Here's how the part is built. I have some questions about the finished solid (model axes, mm). Round coordinates to 2 decimals unless told otherwise and drop trailing zeros. Order: outer loops, then holes, each group sorted by start corner. A loop starts at its lowest first (then second) coordinate and runs counter-clockwise, first axis right, second up. Notation, with made-up numbers: (1, -17.75) -> (53, -17.75) arc R30 cw to (53, 11.25) -> close; hole circle Ø6 at (40, 26.5). An arc over 180 degrees is marked (long way). Use a Markdown table: item, result. Add a question column.
(1) If I drill on probe 1 along Y at (x, z) = (65.5, 55), over which ranges is the centre line in solid material (lowest first)?
(2) I want a section at A-A, the plane y = 9.5. Please give me the cut outline in (x, z) (3 decimals), then the cut area to 3 significant figures.
(3) I want a section at C-C, the plane x = 76. Please give me the cut outline in (y, z).
(4) I'm going to push a flat-ended pin straight in: P1, Ø2, axis at y = 3.5, z = -31.5, coming from the -X side. Where does the tip first touch, or does it pass through?
(5) I want a section at B-B, the plane z = -35.5. Please give me the cut outline in (x, y), then the cut area to 3 significant figures.
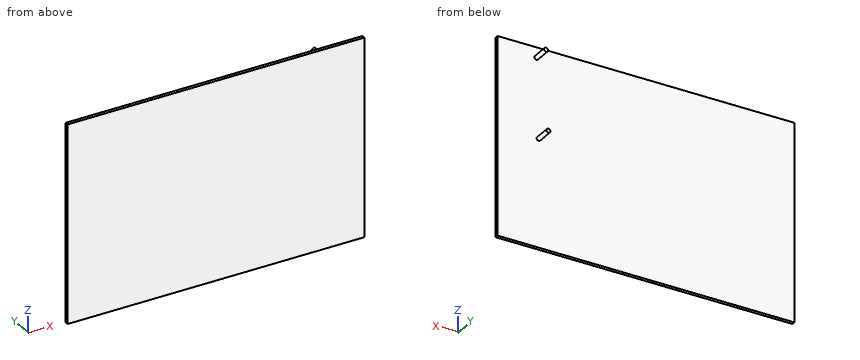
from build123d import *

# Parameters (mm, degrees)
IZIM2_W                     = 180
IZIM2_H                     = 120
Y_KSEKLIK_EKSTR_ZYON1_DEPTH = 2
IZIM3_R                     = 1.225
Y_KSEKLIK_EKSTR_ZYON2_DEPTH = 10


with BuildPart() as part:
    # Çizim2 → Yükseklik-Ekstrüzyon1 (new body)
    with BuildSketch(Plane(origin=(0, 0, 0), x_dir=(1, 0, 0), z_dir=(0, 1, 0))):
        Rectangle(IZIM2_W, IZIM2_H)
    extrude(amount=Y_KSEKLIK_EKSTR_ZYON1_DEPTH)

    # Çizim3 → Yükseklik-Ekstrüzyon2 (add)
    with BuildSketch(Plane(origin=(0, 2, 0), x_dir=(1, 0, 0), z_dir=(0, 1, 0))):
        with Locations(Location((66.5, -53.67, 0), (0, 0, 90))):
            Circle(IZIM3_R)
        with Locations(Location((65.1, -5.37, 0), (0, 0, 90))):
            Circle(IZIM3_R)
    extrude(amount=Y_KSEKLIK_EKSTR_ZYON2_DEPTH)


solid = part.part
Taken from the geometry:
| question | item | result |
|---|---|---|
| 1 | probe 1 | y = 0 to 2 |
| 2 | outline | circle Ø2.45 at (65.1, 5.37); circle Ø2.45 at (66.5, 53.67) |
| 2 | area | 9.43 mm2 |
| 3 | outline | (0, -60) -> (2, -60) -> (2, 60) -> (0, 60) -> close |
| 4 | P1 | passes through |
| 5 | outline | (-90, 0) -> (90, 0) -> (90, 2) -> (-90, 2) -> close |
| 5 | area | 360 mm2 |
